Check sheet for the modelled part. Datum: model origin and axes. Units: mm. A direction names the side the tool comes from. Give positions to 0.01 mm unless a question says otherwise; leave off trailing zeros. Order: outer loops, then holes, each group sorted by start corner. A loop starts at its lowest first (then second) coordinate and runs counter-clockwise, first axis right, second up. Notation, with made-up numbers: (53.5, 42) -> (63.5, 42) arc R7 ccw to (63.5, 55) -> close; hole circle Ø10 at (26, 24). An arc over 180 degrees is marked (long way). Answer in a Markdown table with one row per item. Add a question column.
(1) Set-up check for faces 1 (the face through (0, 6, 1)), 2 (the face through (-2, 6, 8.5)), 3 (the face through (2.285, 3.584, 4.782)): record each of +Z, -Z, +X, -X, +Y, -Y from which the full face is reachable in a straight line by a thin tool's end or side.
(2) Cross-section at B-B (y = -7). Record the cut outline in (x, z), then the cut area to 3 significant figures.
(3) Cross-section at D-D (x = 2.25). Record the cut outline in (y, z), then the cut area to 3 significant figures.
(4) Go/stop test with flat-tipped pins: pin 1 (0.6 mm diameter, centred on x = 4, y = -5, fed in from -Z); pin 2 (5 mm diameter, centred on y = 3, z = 8, fed in from -X); pin 3 (5 mm diameter, centred on x = -3, z = 4.5, fed in from -Y). Record where each tip stops, or that it passes through.
(5) Thickness scan on L1, parallel to Y at x = 0, z = 0.35 (3 decimals); L2, parallel to Z at x = -4.75, y = -5.5; L3, parallel to X at y = -2.25, z = 2. Record the ranges inside material, lowest first. Write a range as [from, to].
(6) Cross-section at A-A (x = 0). Record the cut outline in (y, z) (3 decimals), then the cut area to 4 significant figures.
(7) Cross-section at C-C (z = 0.5). Record the cut outline in (x, y) (3 decimals), then the cut area to 3 significant figures.
(8) Release check for a two-part mould opening along Z. For faces 4 (the face through (-4, -5, 1)), 5 (the face through (-5.723, -1.802, 4.799)), 6 (the face through (-1.73, -7.81, 0.59)) record: released by +Z, released by -Z, zero draft, split by the parting line, or undercut.
```python
from build123d import *

# Parameters (mm, degrees)
SKETCH2_R               = 8
SKETCH2_R_2             = 4.25
BOSS_EXTRUDE1_DEPTH     = 16
SKETCH3_OUTSIDE_W       = 23.542
SKETCH3_OUTSIDE_H       = 23.542
SKETCH3_OUTSIDE_R       = 6
CUT_EXTRUDE1_DEPTH      = 7.3
CUT_EXTRUDE2_REACH      = 26
CUT_EXTRUDE2_END_RADIUS = 4.25
SKETCH6_R               = 1.75
CUT_EXTRUDE3_REACH      = 26
CUT_EXTRUDE3_END_RADIUS = 4.25
SKETCH5_R               = 1.75
CUT_EXTRUDE4_START      = -5.75
SKETCH7_R               = 8
CUT_EXTRUDE4_DEPTH      = 5.75
CUT_EXTRUDE5_START      = -0.55
SKETCH9_R               = 8
CUT_EXTRUDE5_DEPTH      = 0.55
SKETCH10_R              = 1
CUT_EXTRUDE6_DEPTH      = 1


with BuildPart() as part:
    # Sketch2 → Boss-Extrude1 (new body)
    with BuildSketch(Plane.XY):
        Circle(SKETCH2_R)
        Circle(SKETCH2_R_2, mode=Mode.SUBTRACT)
    extrude(amount=BOSS_EXTRUDE1_DEPTH)

    # Sketch3 outside → Cut-Extrude1 (cut)
    with BuildSketch(Plane.XY.offset(1.2)):
        Rectangle(SKETCH3_OUTSIDE_W, SKETCH3_OUTSIDE_H)
        with Locations(Location((0, 0, 0), (0, 0, 180))):
            Circle(SKETCH3_OUTSIDE_R, mode=Mode.SUBTRACT)
    extrude(amount=CUT_EXTRUDE1_DEPTH, mode=Mode.SUBTRACT)

    # Cut-Extrude2: up to this cylinder (the profile starts outside it)
    cut_extrude2_end = Plane(origin=(0, 0, 12.25), z_dir=(0, 0, -1)) * Cylinder(CUT_EXTRUDE2_END_RADIUS, 61.5, mode=Mode.PRIVATE)
    # Sketch6 → Cut-Extrude2 (cut, up to the surface)
    with BuildSketch(Plane(origin=(8, 0, 0), x_dir=(0, 0, -1), z_dir=(1, 0, 0)), mode=Mode.PRIVATE) as cut_extrude2_sk1:
        with Locations((-12.25, 0)):
            Circle(SKETCH6_R)
    cut_extrude2_tool1 = extrude(cut_extrude2_sk1.sketch, amount=-CUT_EXTRUDE2_REACH, mode=Mode.PRIVATE) - cut_extrude2_end
    add(cut_extrude2_tool1.solids().sort_by_distance((8, 0, 12.25))[0], mode=Mode.SUBTRACT)

    # Cut-Extrude3: up to this cylinder (the profile starts outside it)
    cut_extrude3_end = Plane(origin=(0, 0, 12.25), z_dir=(0, 0, -1)) * Cylinder(CUT_EXTRUDE3_END_RADIUS, 61.5, mode=Mode.PRIVATE)
    # Sketch5 → Cut-Extrude3 (cut, up to the surface)
    with BuildSketch(Plane(origin=(0, 8, 0), x_dir=(1, 0, 0), z_dir=(0, 1, 0)), mode=Mode.PRIVATE) as cut_extrude3_sk1:
        with Locations(Location((0, -12.25, 0), (0, 0, 270))):
            Circle(SKETCH5_R)
    cut_extrude3_tool1 = extrude(cut_extrude3_sk1.sketch, amount=-CUT_EXTRUDE3_REACH, mode=Mode.PRIVATE) - cut_extrude3_end
    add(cut_extrude3_tool1.solids().sort_by_distance((0, 8, 12.25))[0], mode=Mode.SUBTRACT)

    # Sketch7 → Cut-Extrude4 (cut)
    with BuildSketch(Plane.XY.offset(16).offset(CUT_EXTRUDE4_START)):
        Circle(SKETCH7_R)
    extrude(amount=CUT_EXTRUDE4_DEPTH, mode=Mode.SUBTRACT)

    # Sketch9 → Cut-Extrude5 (cut)
    with BuildSketch(Plane.XY.offset(10.25).offset(CUT_EXTRUDE5_START)):
        Circle(SKETCH9_R)
    extrude(amount=CUT_EXTRUDE5_DEPTH, mode=Mode.SUBTRACT)

    # Sketch10 → Cut-Extrude6 (cut)
    with BuildSketch(Plane(origin=(0, 0, 0), x_dir=(-1, 0, 0), z_dir=(0, 0, -1))):
        with Locations((0, 6.125)):
            Circle(SKETCH10_R)
        with Locations((5.825221162, 1.892729091)):
            Circle(SKETCH10_R)
        with Locations((3.60018467, -4.955229091)):
            Circle(SKETCH10_R)
        with Locations((-3.60018467, -4.955229091)):
            Circle(SKETCH10_R)
        with Locations((-5.825221162, 1.892729091)):
            Circle(SKETCH10_R)
    extrude(amount=-CUT_EXTRUDE6_DEPTH, mode=Mode.SUBTRACT)


solid = part.part
```
Answer below:
| question | item | result |
|---|---|---|
| 1 | face 1 | -Z |
| 1 | face 2 | none |
| 1 | face 3 | +Z, -Z |
| 2 | outline | (-3.87, 0) -> (3.87, 0) -> (3.87, 1.2) -> (-3.87, 1.2) -> close; (-3.87, 8.5) -> (3.87, 8.5) -> (3.87, 9.7) -> (-3.87, 9.7) -> close |
| 2 | area | 18.6 mm² |
| 3 | outline | (-7.68, 0) -> (-3.61, 0) -> (-3.61, 9.7) -> (-7.68, 9.7) -> (-7.68, 8.5) -> (-5.56, 8.5) -> (-5.56, 1.2) -> (-7.68, 1.2) -> close; (3.61, 0) -> (7.68, 0) -> (7.68, 1.2) -> (5.56, 1.2) -> (5.56, 8.5) -> (7.68, 8.5) -> (7.68, 9.7) -> (3.61, 9.7) -> close |
| 3 | area | 48.1 mm² |
| 4 | pin 1 | stops at z = 1 |
| 4 | pin 2 | stops at x = -7.98 |
| 4 | pin 3 | stops at y = -5.98 |
| 5 | L1 | y = [-8, -4.25], [4.25, 5.125], [7.125, 8] |
| 5 | L2 | z = [0, 1.2], [8.5, 9.7] |
| 5 | L3 | x = [-5.56, -3.61], [3.61, 5.56] |
| 6 | outline | (-8, 0) -> (-4.25, 0) -> (-4.25, 9.7) -> (-8, 9.7) -> (-8, 8.5) -> (-6, 8.5) -> (-6, 1.2) -> (-8, 1.2) -> close; (4.25, 0) -> (5.125, 0) -> (5.125, 1) -> (7.125, 1) -> (7.125, 0) -> (8, 0) -> (8, 1.2) -> (6, 1.2) -> (6, 8.5) -> (8, 8.5) -> (8, 9.7) -> (4.25, 9.7) -> close |
| 6 | area | 41.55 mm² |
| 7 | outline | circle Ø16 at (0, 0); hole circle Ø2 at (-5.825, 1.893); hole circle Ø2 at (-3.6, -4.955); hole circle Ø8.5 at (0, 0); hole circle Ø2 at (0, 6.125); hole circle Ø2 at (3.6, -4.955); hole circle Ø2 at (5.825, 1.893) |
| 7 | area | 129 mm² |
| 8 | face 4 | released by -Z |
| 8 | face 5 | undercut |
| 8 | face 6 | zero draft |
